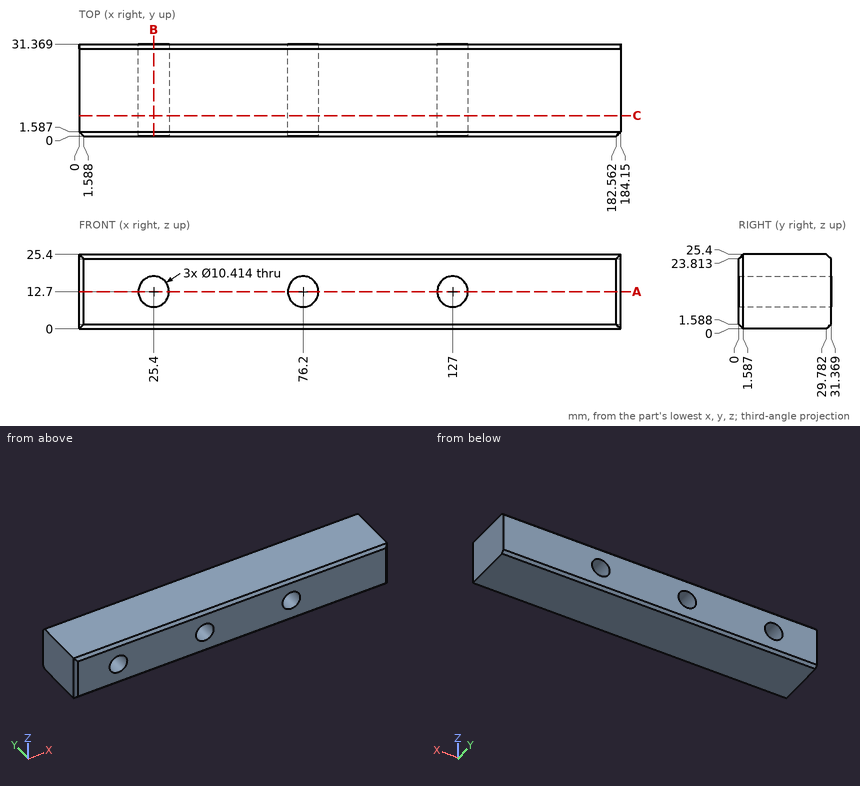
Drawing for the job (mm, zero at the part's lowest x, y, z). Round coordinates to 2 decimals unless told otherwise and drop trailing zeros. Write each loop counter-clockwise with the first axis right and the second up, starting at its lowest first coordinate (ties: lowest second). Pieces come first, ordered by that corner, then holes.
Item 1: Band-saw the part on B-B on x = 25.4. Write the cut outline in (y, z).
Filled in:
outline: (0, 1.59) - (1.59, 0) - (29.78, 0) - (31.37, 1.59) - (31.37, 7.49) - (0, 7.49) - close; (0, 17.91) - (31.37, 17.91) - (31.37, 23.81) - (29.78, 25.4) - (1.59, 25.4) - (0, 23.81) - close
Item 2: Band-saw the part on C-C on y = 7. Give the number of separate pieces and of enclosed holes in the cut face, then the cut area to 3 significant figures.
Filled in:
separate pieces: 1
enclosed holes: 3
area: 4,420 mm2
Item 3: Drill centre lines: L1, parallel to X at y = 10, z = 14; L2, parallel to X at y = 16.5, z = 16.25; L3, parallel to Z at x = 76, y = 8. Where is each one in solid material? Low to high.
Filled in:
L1: x = 0 to 20.36, 30.44 to 71.16, 81.24 to 121.96, 132.04 to 184.15
L2: x = 0 to 21.59, 29.21 to 72.39, 80.01 to 123.19, 130.81 to 184.15
L3: z = 0 to 7.5, 17.9 to 25.4
Item 4: Band-saw the part on A-A on z = 12.7. Write the cut outline in (x, y).
Filled in:
outline: (0, 1.59) - (1.59, 0) - (20.19, 0) - (20.19, 31.37) - (0, 31.37) - close; (30.61, 0) - (70.99, 0) - (70.99, 31.37) - (30.61, 31.37) - close; (81.41, 0) - (121.79, 0) - (121.79, 31.37) - (81.41, 31.37) - close; (132.21, 0) - (182.56, 0) - (184.15, 1.59) - (184.15, 31.37) - (132.21, 31.37) - close
